Geometry check sheet. Reference: the model listing, model coordinates, mm. A direction names the side the tool comes from. Coordinates: 2 decimals unless noted, no trailing zeros. Order: outer loops, then holes, each group sorted by start corner. A loop starts at its lowest first (then second) coordinate and runs counter-clockwise, first axis right, second up.
```python
from build123d import *

# Parameters (mm, degrees)
SKETCH1_W           = 406.4
SKETCH1_H           = 25.4
BOSS_EXTRUDE1_DEPTH = 25.4
SHELL1_T            = -3.175


with BuildPart() as part:
    # Sketch1 → Boss-Extrude1 (new body, symmetric)
    with BuildSketch(Plane(origin=(0, 0, 0), x_dir=(1, 0, 0), z_dir=(0, 1, 0))):
        Rectangle(SKETCH1_W, SKETCH1_H)
    extrude(amount=BOSS_EXTRUDE1_DEPTH, both=True)

    # Shell1
    shell1_openings = [part.faces().sort_by_distance(p)[0] for p in [
        (-203.2, 0, 0),
        (203.2, 0, 0),
    ]]
    offset(amount=SHELL1_T, openings=shell1_openings, kind=Kind.INTERSECTION)


solid = part.part
```
Item 1: Sectioned sample at A-A (z = -1.75). Record the cut outline in (x, y) (3 decimals), and give its area (3 significant figures).
Item 2: Sectioned sample at C-C (x = -147). Record the cut outline in (y, z) (3 decimals), and give its area (3 significant figures).
Item 3: Depth check by flat-ended pin: P1, Ø4, axis at y = 3, z = 6, coming from the -X side; P2, Ø1, axis at y = -15.5, z = 9.5, coming from the -X side. Enter the tip coordinate at first touch or a pass-through.
Item 4: Tool access check on faces 1 (the face through (-3, 0, 9.525)), 2 (the face through (-3, 0, -12.7)). Record the directions out of +Z, -Z, +X, -X, +Y, -Y that give a thin tool (end or side, any length) a straight path to the whole face; none if there is none.
Item 5: Release check for a two-part mould opening along Y. For faces 3 (the face through (-3, 22.225, 0)), 4 (the face through (-203.2, -2, 10)), 5 (the face through (-3, 25.4, 0)), 6 (the face through (-3, -22.225, 0)) record: pulls with the +Y half, pulls with the -Y half, needs draft (parallel to the pull), parting line crosses it, or undercut.
Item 6: Sectioned sample at B-B (y = 11.5). Record the cut outline in (x, z) (3 decimals).
Item 7: Thickness scan on line 1 along Z through (x, y) = (128, 5) (3 decimals); line 2 along Y through (x, z) = (38.5, -1.5) (3 decimals). Record the ranges inside material, lowest first.
Geometry check:
1. outline: (-203.2, -25.4) - (203.2, -25.4) - (203.2, -22.225) - (-203.2, -22.225) - close; (-203.2, 22.225) - (203.2, 22.225) - (203.2, 25.4) - (-203.2, 25.4) - close
1. area: 2,580 mm2
2. outline: (-25.4, -12.7) - (25.4, -12.7) - (25.4, 12.7) - (-25.4, 12.7) - close; hole (-22.225, -9.525) - (22.225, -9.525) - (22.225, 9.525) - (-22.225, 9.525) - close
2. area: 444 mm2
3. P1: passes through
3. P2: stops at x = -203.2
4. face 1: +X, -X
4. face 2: -Z, +X, -X, +Y, -Y
5. face 3: undercut
5. face 4: needs draft
5. face 5: pulls with the +Y half
5. face 6: undercut
6. outline: (-203.2, -12.7) - (203.2, -12.7) - (203.2, -9.525) - (-203.2, -9.525) - close; (-203.2, 9.525) - (203.2, 9.525) - (203.2, 12.7) - (-203.2, 12.7) - close
7. line 1: z = -12.7 to -9.525, 9.525 to 12.7
7. line 2: y = -25.4 to -22.225, 22.225 to 25.4
